Can you work these out from the model? Positions are in its coordinate system, mm. A direction names the side the tool comes from. Give positions to 0.01 mm unless a question says otherwise; leave off trailing zeros. Order: outer loops, then holes, each group sorted by start corner. A loop starts at its lowest first (then second) coordinate and runs counter-clockwise, first axis right, second up. Notation, with made-up numbers: (58, 44) - (87, 44) arc R25 cw to (87, 59) - close; hole circle Ø10 at (59.25, 6). An arc over 180 degrees is marked (long way). Answer as a JSON object with one key per item and string values.
```python
from build123d import *

# Parameters (mm, degrees)
EXTRUDE_1_DEPTH              = 3
CUT_EXTRUDE_START            = 3
CUT_EXTRUDE_2_DEPTH          = 1
CUT_EXTRUDE_3_DEPTH          = 136.739649697
CUT_EXTRUDE_3_DEPTH_BACK     = 136.739649697
HOLE_WIZARD_M3_1_D           = 3.2
HOLE_WIZARD_M3_1_CSINK_D     = 6.3
HOLE_WIZARD_M3_1_CSINK_ANGLE = 90
M4X0_7_1_D                   = 3.3
M3X0_5_1_D                   = 3
PATTERN_LINEAR_1_COUNT       = 8
PATTERN_LINEAR_1_PITCH       = 30


with BuildPart() as part:
    # ｽｹｯﾁ1 → ﾎﾞｽ - 押し出し1 (new, symmetric)
    with BuildSketch(Plane.XY):
        with BuildLine():
            Line((-122.45, 58.5), (122.45, 58.5))
            Line((122.45, 58.5), (122.45, 11.5))
            Line((122.45, 11.5), (67.187698744, 11.5))
            ThreePointArc((67.187698744, 11.5), (66.687698744, 12), (66.187698744, 11.5))
            Line((66.187698744, 11.5), (66.187698744, -48.5))
            Line((66.187698744, -48.5), (-66.187698744, -48.5))
            Line((-66.187698744, -48.5), (-66.187698744, 11.5))
            ThreePointArc((-66.187698744, 11.5), (-66.687698744, 12), (-67.187698744, 11.5))
            Line((-67.187698744, 11.5), (-122.45, 11.5))
            Line((-122.45, 11.5), (-122.45, 58.5))
        make_face()
    extrude(amount=EXTRUDE_1_DEPTH, both=True)

    # ｽｹｯﾁ1<4> → ｶｯﾄ - 押し出し2 (cut)
    with BuildSketch(Plane.XY.offset(CUT_EXTRUDE_START)):
        with BuildLine():
            Line((-116.45, 58.5), (-122.45, 58.5))
            Line((-122.45, 58.5), (-122.45, 11.5))
            Line((-122.45, 11.5), (-67.187698744, 11.5))
            ThreePointArc((-67.187698744, 11.5), (-66.687698744, 12), (-66.187698744, 11.5))
            Line((-66.187698744, 11.5), (-66.187698744, -48.5))
            Line((-66.187698744, -48.5), (66.187698744, -48.5))
            Line((66.187698744, -48.5), (66.187698744, 11.5))
            ThreePointArc((66.187698744, 11.5), (66.687698744, 12), (67.187698744, 11.5))
            Line((67.187698744, 11.5), (122.45, 11.5))
            Line((122.45, 11.5), (122.45, 58.5))
            Line((122.45, 58.5), (116.45, 58.5))
            Line((116.45, 58.5), (116.45, 17.5))
            Line((116.45, 17.5), (66.187698744, 17.5))
            Line((66.187698744, 17.5), (66.187698744, 18.5))
            ThreePointArc((66.187698744, 18.5), (65.687698744, 19), (65.187698744, 18.5))
            Line((65.187698744, 18.5), (61.187698744, 18.5))
            ThreePointArc((61.187698744, 18.5), (60.687698744, 19), (60.187698744, 18.5))
            Line((60.187698744, 18.5), (60.187698744, -42.5))
            Line((60.187698744, -42.5), (-60.187698744, -42.5))
            Line((-60.187698744, -42.5), (-60.187698744, 18.5))
            ThreePointArc((-60.187698744, 18.5), (-60.687698744, 19), (-61.187698744, 18.5))
            Line((-61.187698744, 18.5), (-65.187698744, 18.5))
            ThreePointArc((-65.187698744, 18.5), (-65.687698744, 19), (-66.187698744, 18.5))
            Line((-66.187698744, 18.5), (-66.187698744, 17.5))
            Line((-66.187698744, 17.5), (-116.45, 17.5))
            Line((-116.45, 17.5), (-116.45, 58.5))
        make_face()
    extrude(amount=-CUT_EXTRUDE_2_DEPTH, mode=Mode.SUBTRACT)

    # ｽｹｯﾁ1<5> → ｶｯﾄ - 押し出し3 (cut, two sides: drawn at the far end of the back side and taken through both)
    with BuildSketch(Plane.XY.offset(-CUT_EXTRUDE_3_DEPTH_BACK)):
        with BuildLine():
            Line((-37, 16.5), (37, 16.5))
            ThreePointArc((37, 16.5), (37.353553391, 16.353553391), (37.5, 16))
            Line((37.5, 16), (37.5, -28))
            ThreePointArc((37.5, -28), (37.353553391, -28.353553391), (37, -28.5))
            Line((37, -28.5), (-37, -28.5))
            ThreePointArc((-37, -28.5), (-37.353553391, -28.353553391), (-37.5, -28))
            Line((-37.5, -28), (-37.5, 16))
            ThreePointArc((-37.5, 16), (-37.353553391, 16.353553391), (-37, 16.5))
        make_face()
    extrude(amount=CUT_EXTRUDE_3_DEPTH + CUT_EXTRUDE_3_DEPTH_BACK, mode=Mode.SUBTRACT)

    # M3 丸皿ねじ用皿穴1 (through all)
    with Locations(Plane(origin=(119.45, 48.5, -3), x_dir=(-1, 0, 0), z_dir=(0, 0, -1))):
        with Locations((0, 0), (0, -28), (11, -34), (45.262301256, -34), (56.262301256, -39.5), (56.262301256, -64), (56.262301256, -88.5), (74.45, -94), (104.45, -94), (134.45, -94), (164.45, -94), (182.637698744, -88.5), (182.637698744, -64), (182.637698744, -39.5), (193.637698744, -34), (227.9, -34), (238.9, -28), (238.9, 0)):
            CounterSinkHole(HOLE_WIZARD_M3_1_D / 2, HOLE_WIZARD_M3_1_CSINK_D / 2, counter_sink_angle=HOLE_WIZARD_M3_1_CSINK_ANGLE)

    # ｽｹｯﾁ4 → M3x0.5 ねじ穴2 (revolve, cut)
    with BuildSketch(Plane(origin=(-105, 58.5, 0), x_dir=(0, 0, 1), z_dir=(1, 0, 0))):
        Polygon((0, 0), (0, 9.251075774), (1.25, 8.5), (1.25, 6), (1.5, 6), (1.5, 0), align=None)
    m3x0_5_2 = revolve(axis=Axis((-105, 64.85, 0), (0, -1, 0)), mode=Mode.SUBTRACT)

    # M4x0.7 ねじ穴1 (through all)
    with Locations(Plane(origin=(42, 19, -3), x_dir=(-1, 0, 0), z_dir=(0, 0, -1))):
        with Locations((0, 0), (84, 0), (84, -50), (0, -50)):
            Hole(M4X0_7_1_D / 2)

    # M3x0.5 ねじ穴1 (through all)
    with Locations(Plane(origin=(-80, 50, 3), x_dir=(1, 0, 0), z_dir=(0, 0, 1))):
        with Locations((0, 0), (160, 0)):
            Hole(M3X0_5_1_D / 2)

    # 直線ﾊﾟﾀｰﾝ1: M3x0.5 ねじ穴2 ×8
    with Locations(*[(i * PATTERN_LINEAR_1_PITCH, 0, 0) for i in range(1, PATTERN_LINEAR_1_COUNT)]):
        add(m3x0_5_2, mode=Mode.SUBTRACT)


solid = part.part
```
Q1. I need wall thicknesses on L1, parallel to X at y = -45.5, z = 0.2; L2, parallel to X at y = -40, z = 0.85; L3, parallel to X at y = 14.5, z = 0.75. Which ranges of each line are inside material? Lowest first, please.
Recorded:
{"L1": "x = -66.19 to -46.6, -43.4 to -16.6, -13.4 to 13.4, 16.6 to 43.4, 46.6 to 66.19", "L2": "x = -66.19 to -64.79, -61.59 to 61.59, 64.79 to 66.19", "L3": "x = -122.45 to -110.05, -106.85 to -75.79, -72.59 to -37.5, 37.5 to 72.59, 75.79 to 106.85, 110.05 to 122.45"}
Q2. If we section it at C-C, the plane x = 88: Please give me the cut outline in (y, z).
Recorded:
{"outline": "(11.5, -3) - (58.5, -3) - (58.5, 3) - (17.5, 3) - (17.5, 2) - (11.5, 2) - close"}
Q3. Which directions (+Z, -Z, +X, -X, +Y, -Y) give clear straight access to the entire face, cutting with the end or side of a thin tool? Please do faces 1 (the face through (-94, 11.5, 0)), 2 (the face through (-122.45, 35, 0)), 3 (the face through (95, 11.5, 0)), 4 (the face through (1, -28.5, 0)).
Recorded:
{"face 1": "+Z, -Z, -X, -Y", "face 2": "+Z, -Z, -X, +Y, -Y", "face 3": "+Z, -Z, +X, -Y", "face 4": "+Z, -Z"}
Q4. I'm going to push flat-ended pins straight in: pin 1 Ø3.5 at (x, y) = (108.45, 14.5) entering from +Z; pin 2 Ø2.5 at (y, z) = (-20, -1) entering from +X; pin 3 Ø5 at (x, y) = (63.19, -15.5) entering from -Z. Where does each tip first touch, or does it pass through?
Recorded:
{"pin 1": "stops at z = 2", "pin 2": "stops at x = 66.19", "pin 3": "stops at z = -2.35"}
Q5. We'd pull the mould along X, two halves only. Please class faces 5 (the face through (-66.188, -19, 0)), 6 (the face through (37.5, -6, 0)), 7 (the face through (1, -48.5, 0)): released by +X, released by -X, zero draft, split by the parting line, or undercut.
Recorded:
{"face 5": "released by -X", "face 6": "undercut", "face 7": "zero draft"}
Q6. If we section it at B-B, the plane x = 21.5: Please give me the cut outline in (y, z).
Recorded:
{"outline": "(-48.5, -3) - (-28.5, -3) - (-28.5, 3) - (-42.5, 3) - (-42.5, 2) - (-48.5, 2) - close; (16.5, -3) - (58.5, -3) - (58.5, 3) - (16.5, 3) - close"}
Q7. If we section it at A-A, the plane y = -10: Please give me the cut outline in (x, z).
Recorded:
{"outline": "(-66.19, -3) - (-37.5, -3) - (-37.5, 3) - (-60.19, 3) - (-60.19, 2) - (-66.19, 2) - close; (37.5, -3) - (66.19, -3) - (66.19, 2) - (60.19, 2) - (60.19, 3) - (37.5, 3) - close"}
